Job drawing, mm, ordinate dimensions from the low corner. One solid piece. Give positions to 0.01 mm unless a question says otherwise; leave off trailing zeros. Loops run counter-clockwise (first coordinate to the right, second up) from the corner with the lowest first, then second, coordinate; pieces in that order, holes last.
Item 1: Mould opens along X. For the marked faces 1, 2, 3 and 4 say: released by +X, released by -X, zero draft, split by the parting line, or undercut.
Item 2: Saw through at A-A on z = 270. Give the cut face in (x, y), plus the area to 3 significant figures.
Item 3: Drop flat-ended pins along their axis: P1, Ø1.5, axis at x = 65, z = 90, coming from the -Y side; P2, Ø4, axis at x = 60.5, y = 90.5, coming from the +Z side; P3, Ø3, axis at x = 133.5, y = 42, coming from the -Z side. Give the stop position or say it passes through.
Item 4: Probe probe 1 along Y at (x, z) = (87, 63); probe 2 along Z at (x, y) = (58, 84); probe 3 along Z at (x, y) = (132.5, 60.5). List the from-to ranges inside material, lowest first.
Item 5: Saw through at B-B on x = 243. Give the cut face in (y, z), plus the area to 3 significant figures.
Item 6: Saw through at C-C on y = 94.5. Give the cut face in (x, z), plus the area to 3 significant figures.
Item 7: Saw through at D-D on z = 90. Give the cut face in (x, y), plus the area to 3 significant figures.
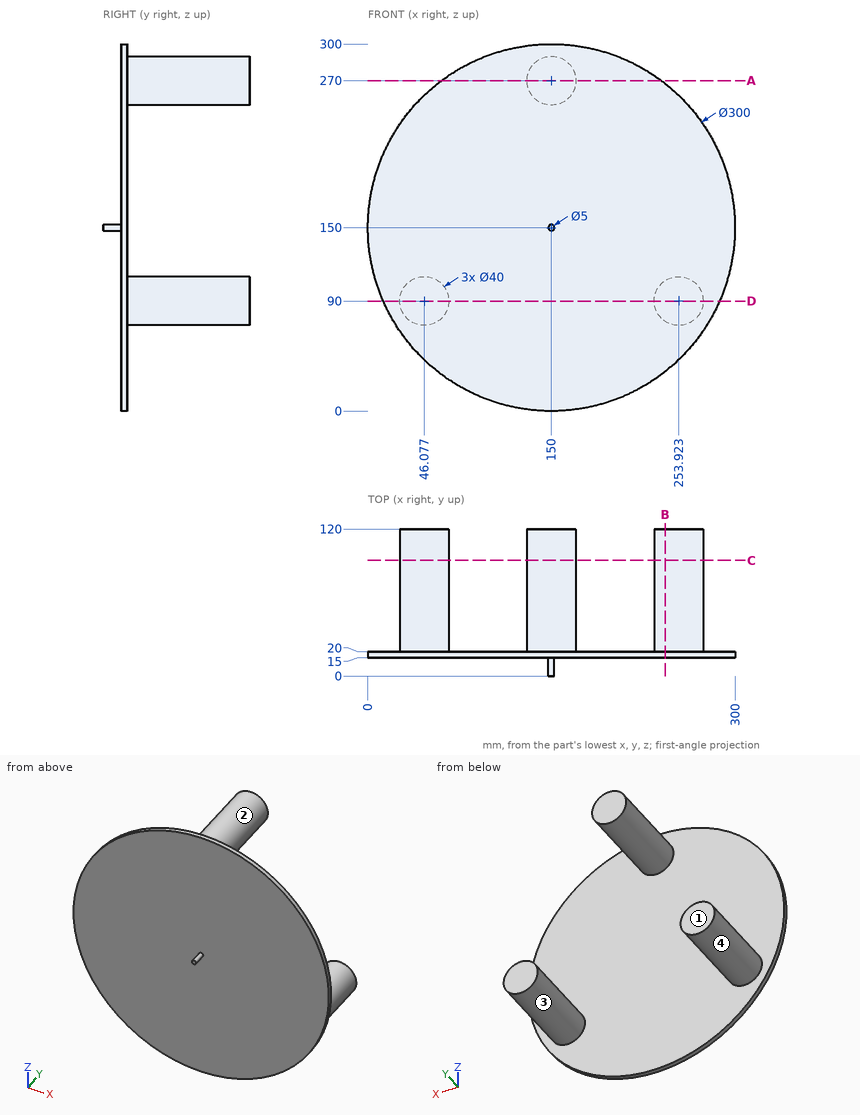
Results below:
1. face 1: zero draft
1. face 2: split by the parting line
1. face 3: undercut
1. face 4: undercut
2. outline: (60, 15) - (240, 15) - (240, 20) - (170, 20) - (170, 120) - (130, 120) - (130, 20) - (60, 20) - close
2. area: 4,900 mm2
3. P1: stops at y = 15
3. P2: stops at z = 105.67
3. P3: stops at z = 256.77
4. probe 1: y = 15 to 20
4. probe 2: z = 73.94 to 106.06
4. probe 3: z = 260.32 to 279.68
5. outline: (15, 32.31) - (20, 32.31) - (20, 73.25) - (120, 73.25) - (120, 106.75) - (20, 106.75) - (20, 267.69) - (15, 267.69) - close
5. area: 4,530 mm2
6. outline: circle Ø40 at (46.08, 90); circle Ø40 at (150, 270); circle Ø40 at (253.92, 90)
6. area: 3,770 mm2
7. outline: (12.52, 15) - (287.48, 15) - (287.48, 20) - (273.92, 20) - (273.92, 120) - (233.92, 120) - (233.92, 20) - (66.08, 20) - (66.08, 120) - (26.08, 120) - (26.08, 20) - (12.52, 20) - close
7. area: 9,370 mm2
